```python
from build123d import *

# Parameters (mm, degrees)
SKETCH001_R             = 30
PAD001_DEPTH            = 12
SKETCH002_R             = 22.5
PAD002_DEPTH            = 14
SKETCH003_R             = 21.5
PAD003_DEPTH            = 10
SKETCH004_R             = 1.5
PAD004_DEPTH            = 10
SKETCH005_R             = 2.5
PAD005_DEPTH            = 10
BODY001_PLACEMENT_ANGLE = 90


with BuildPart() as part:
    # Sketch001 → Pad001 (new body)
    with BuildSketch(Plane.XY):
        Circle(SKETCH001_R)
    extrude(amount=PAD001_DEPTH)

    # Sketch002 (on Face3 of Pad001) → Pad002 (join)
    with BuildSketch(Plane.XY.offset(12)):
        Circle(SKETCH002_R)
    extrude(amount=PAD002_DEPTH)

    # Sketch003 (on Face2 of Pad002) → Pad003 (join)
    with BuildSketch(Plane(origin=(0, 0, 0), x_dir=(1, 0, 0), z_dir=(0, 0, -1))):
        Circle(SKETCH003_R)
    extrude(amount=PAD003_DEPTH)

    # Sketch004 (on Face2 of Pad003) → Pad004 (join)
    with BuildSketch(Plane(origin=(0, 0, 0), x_dir=(1, 0, 0), z_dir=(0, 0, -1))):
        with Locations((0, 25)):
            Circle(SKETCH004_R)
        with Locations((21.65, -12.5)):
            Circle(SKETCH004_R)
        with Locations((-21.65, -12.5)):
            Circle(SKETCH004_R)
    extrude(amount=PAD004_DEPTH)

    # Sketch005 (on Face13 of Pad004) → Pad005 (join)
    with BuildSketch(Plane.XY.offset(26)):
        with Locations((8, 15)):
            Circle(SKETCH005_R)
    extrude(amount=PAD005_DEPTH)


with BuildPart() as part_1:
    # Body001 placement: moved
    add(part.part.moved(Location((0, 0, 70))).rotate(Axis((0, 0, 70), (1, 0, 0)), BODY001_PLACEMENT_ANGLE))


solid = part_1.part
```
Could you check a few things on this model? Use its own coordinates, in mm. A direction names the side the tool comes from. Round coordinates to 2 decimals unless told otherwise and drop trailing zeros. Order: outer loops, then holes, each group sorted by start corner. A loop starts at its lowest first (then second) coordinate and runs counter-clockwise, first axis right, second up. Notation, with made-up numbers: (80, 87.25) -> (112, 87.25) arc R26 ccw to (112, 118.25) -> close; hole circle Ø2 at (-38, 41.25). An arc over 180 degrees is marked (long way). One line per question, with ' | ' between items.
Q1. If we section it at A-A on y = 4: Write out the boundary of the cut face in (x, z), plus the area to 3 significant figures.
Computed values:
outline: circle Ø3 at (-21.65, 82.5); circle Ø43 at (0, 70); circle Ø3 at (0, 45); circle Ø3 at (21.65, 82.5) | area: 1,470 mm²
Q2. Which directions (+Z, -Z, +X, -X, +Y, -Y) give clear straight access to the entire face, cutting with the end or side of a thin tool? Please do faces 1 (the face through (4.3, -12, 92.4)), 2 (the face through (9, 0, 50)), 3 (the face through (8, -36, 85)).
Computed values:
face 1: -Y | face 2: +Y | face 3: +Z, -Z, +X, -X, -Y
Q3. If I drill on line 1 (Y direction, x = 28.5, z = 70.5); line 2 (Y direction, x = 13, z = 57.5); line 3 (Z direction, x = -12.5, y = -13.5), over which ranges is the centre line in solid material (lowest first)? Write a range as from..to.
Computed values:
line 1: -12..0 | line 2: -26..10 | line 3: 51.29..88.71
Q4. If we section it at C-C on z = 70: Write out the boundary of the cut face in (x, y).
Computed values:
outline: (-30, -12) -> (-22.5, -12) -> (-22.5, -26) -> (22.5, -26) -> (22.5, -12) -> (30, -12) -> (30, 0) -> (21.5, 0) -> (21.5, 10) -> (-21.5, 10) -> (-21.5, 0) -> (-30, 0) -> close
Q5. We'd pull the mould along Z, two halves only. Please class faces 4 (the face through (22, 10, 82)), 5 (the face through (22.456, 4.93, 81.235)), 6 (the face through (-22.76, 4.93, 81.49)), 7 (the face through (-2.93, -18.9, 92.31)): released by +Z, released by -Z, zero draft, split by the parting line, or undercut.
Computed values:
face 4: zero draft | face 5: undercut | face 6: undercut | face 7: split by the parting line
Q6. If we section it at B-B on x = 0: Write out the boundary of the cut face in (y, z), plus the area to 3 significant figures.
Computed values:
outline: (-26, 47.5) -> (-12, 47.5) -> (-12, 40) -> (0, 40) -> (0, 43.5) -> (10, 43.5) -> (10, 46.5) -> (0, 46.5) -> (0, 48.5) -> (10, 48.5) -> (10, 91.5) -> (0, 91.5) -> (0, 100) -> (-12, 100) -> (-12, 92.5) -> (-26, 92.5) -> close | area: 1,810 mm²
Q7. If we section it at D-D on y = -14: Write out the boundary of the cut face in (x, z), plus the area to 3 significant figures.
Computed values:
outline: circle Ø45 at (0, 70) | area: 1,590 mm²
Q8. I'm going to push flat-ended pins straight in: pin 1 (4 mm diameter, centred on y = -21.5, z = 60.5, fed in from -X); pin 2 (6 mm diameter, centred on x = 1.5, y = -27, fed in from -Z); pin 3 (10 mm diameter, centred on x = 10.5, z = 50, fed in from -Y); pin 4 (10 mm diameter, centred on y = -1, z = 67.5, fed in from -X). Where does each tip first touch, or does it pass through?
Computed values:
pin 1: x = -21.21 | pin 2: z = 47.5 | pin 3: y = -26 | pin 4: x = -30
